The listing builds one solid part. Answer for the finished solid, in the listing's coordinates (mm). A direction names the side the tool comes from. Give positions to 0.01 mm unless a question says otherwise; leave off trailing zeros. Loops run counter-clockwise (first coordinate to the right, second up) from the corner with the lowest first, then second, coordinate; pieces in that order, holes last. Notation, with made-up numbers: (-3.5, 54.25) - (36.5, 54.25) arc R28 ccw to (36.5, 75.25) - close; hole circle Ø7 at (-22.75, 48.5). An arc over 180 degrees is marked (long way). One line per item, written item: value. Start each with the question number.
from build123d import *

# Parameters (mm, degrees)
BOSS_EXTRUDE1_DEPTH = 2.5
BOSS_EXTRUDE2_DEPTH = 10
SKETCH3_R           = 3.1
CUT_EXTRUDE1_DEPTH  = 97.926231277
BOSS_EXTRUDE3_DEPTH = 10
SKETCH5_R           = 3.1
CUT_EXTRUDE2_DEPTH  = 73.924932584
SKETCH6_W           = 5.175957564
SKETCH6_H           = 5
CUT_EXTRUDE3_DEPTH  = 113.454585159


with BuildPart() as part:
    # Sketch1 → Boss-Extrude1 (new body, symmetric)
    with BuildSketch(Plane(origin=(-32.81203924, 33.9517387, -54.90733973), x_dir=(-1, 0, 0), z_dir=(0, -1, 0))):
        Polygon((57.454585159, 35), (-55, 35), (-55, 0.15), (-34.85, 0.15), (-34.85, -5.15), (-55, -5.15), (-55, -85), (57.454585159, -85), (57.454585159, -4.673151813), (37.304585159, -4.673151813), (37.304585159, 0.626848187), (57.454585159, 0.626848187), align=None)
    extrude(amount=BOSS_EXTRUDE1_DEPTH, both=True)

    # Sketch2 → Boss-Extrude2 (add)
    with BuildSketch(Plane.ZY.offset(90.266624399)):
        Polygon((7.48223475, 36.4517387), (19.180938343, 44.643259143), (24.916702706, 36.4517387), align=None)
    boss_extrude2 = extrude(amount=-BOSS_EXTRUDE2_DEPTH)

    # Sketch3 → Cut-Extrude1 (cut, through all)
    with BuildSketch(Plane(origin=(0, 23.699275736, 33.846073404), x_dir=(1, 0, 0), z_dir=(0, 0.573576436, 0.819152044))):
        with Locations((-85.266624399, 19.56788273)):
            Circle(SKETCH3_R)
    cut_extrude1 = extrude(amount=-CUT_EXTRUDE1_DEPTH, mode=Mode.SUBTRACT)

    # Sketch4 → Boss-Extrude3 (add)
    with BuildSketch(Plane(origin=(-70.266624399, 0, 0), x_dir=(0, 0, -1), z_dir=(1, 0, 0))):
        Polygon((76.559676692, 36.4517387), (80.950923398, 42.723088931), (89.90733973, 36.4517387), align=None)
    boss_extrude3 = extrude(amount=-BOSS_EXTRUDE3_DEPTH)

    # Sketch5 → Cut-Extrude2 (cut, through all)
    with BuildSketch(Plane(origin=(0, 66.702115647, -46.70532419), x_dir=(1, 0, 0), z_dir=(0, 0.819152044, -0.573576436))):
        with Locations((-75.266624399, 47.80615729)):
            Circle(SKETCH5_R)
    cut_extrude2 = extrude(amount=-CUT_EXTRUDE2_DEPTH, mode=Mode.SUBTRACT)

    # Mirror1: Boss-Extrude2, Cut-Extrude1, Boss-Extrude3, Cut-Extrude2 across plane
    add(boss_extrude2.mirror(Plane.ZY.offset(34.03933182)))
    add(cut_extrude1.mirror(Plane.ZY.offset(34.03933182)), mode=Mode.SUBTRACT)
    add(boss_extrude3.mirror(Plane.ZY.offset(34.03933182)))
    add(cut_extrude2.mirror(Plane.ZY.offset(34.03933182)), mode=Mode.SUBTRACT)

    # Sketch6 → Cut-Extrude3 (cut, through all)
    with BuildSketch(Plane.ZY.offset(90.266624399)):
        with Locations((27.504681488, 33.9517387)):
            Rectangle(SKETCH6_W, SKETCH6_H)
    extrude(amount=-CUT_EXTRUDE3_DEPTH, mode=Mode.SUBTRACT)


solid = part.part
1. Flat-ended cylindrical pins translate along their axes: pin 1 (7 mm diameter, centred on y = 40.5, z = -80, fed in from +X); pin 2 (4 mm diameter, centred on y = 35, z = -53.5, fed in from -X); pin 3 (3 mm diameter, centred on y = 38.5, z = -86.5, fed in from -X). Find the tip coordinate at first contact, or state that the pin passes through.
2. A cutting plane is placed at A-A (z = -37.5). Determine the outline of the cut face in (x, y).
3. Find the intervals of material crossed by L1, parallel to X at y = 37.25, z = 14; L2, parallel to Y at x = -48, z = -29; L3, parallel to Z at x = 7.5, y = 36.75, in increasing order. Write a range as [from, to].
4. For faces 5 (the flat face through (12.188, 39, -82)), 6 (the flat face through (-70.267, 39, -82)), 7 (the flat face through (-70.117, 34, -53)), determine the directions among +Z, -Z, +X, -X, +Y, -Y from which every point of the face is accessible in a straight line to the end or side of a thin tool.
5. A cutting plane is placed at B-B (x = -52). Determine the outline of the cut face in (y, z), plus the area to 3 significant figures.
6. Determine the mould class of faces 1 (the cylindrical face through (-73.84, 37.19, -81.04)), 2 (the flat face through (-33, 36.452, -33)), 3 (the cylindrical face through (17.592, 38.116, 14.96)), 4 (the flat face through (-35, 34, 24.917)) for opening direction Y: released by +Y, released by -Y, zero draft, split by the parting line, or undercut.
Results below:
1. pin 1: stops at x = 12.19
1. pin 2: stops at x = -70.12
1. pin 3: stops at x = -80.27
2. outline: (-90.27, 31.45) - (22.19, 31.45) - (22.19, 36.45) - (-90.27, 36.45) - close
3. L1: x = [-90.27, -86.32], [-84.21, -80.27], [12.19, 16.13], [18.24, 22.19]
3. L2: y = [31.45, 36.45]
3. L3: z = [-89.48, -87.86], [-80.33, -76.77]
4. face 5: -Z, +X, +Y
4. face 6: +Z, -Z, +Y
4. face 7: -X, +Y, -Y
5. outline: (31.45, -89.91) - (36.45, -89.91) - (36.45, 24.92) - (31.45, 24.92) - close
5. area: 574 mm^2
6. face 1: undercut
6. face 2: released by +Y
6. face 3: undercut
6. face 4: zero draft
